Print and shaded views of the part. All mm, measured from the part's lowest x, y and z. Round coordinates to 2 decimals unless told otherwise and drop trailing zeros. Write each question's results on one line, items separated by ' | '. Start each with the question number.
1. Two-plate mould, pull along X, no slides. Class the marked faces 1, 2, 3 and 4: +X half, -X half, draft (parallel to the pull), parting line (faces both ways), or undercut.
2. Probe L1, parallel to Y at x = 2.5, z = 6; L2, parallel to X at y = 4.75, z = 9.5 (1 decimal); L3, parallel to Z at x = 7.5, y = 10.75 (1 decimal). List the from-to ranges inside material, lowest first. Write a range as [from, to].
3. Band-saw the part on A-A, the plane x = 5. Give the number of separate pieces and of enclosed holes in the cut face, then the cut area to 3 significant figures.
4. Drop flat-ended pins along their axis: pin 1 Ø4 at (x, y) = (5.5, 25.5) entering from -Z; pin 2 Ø1 at (x, z) = (5.5, 8.5) entering from +Y; pin 3 Ø3.5 at (x, y) = (5, 4.98) entering from -Z. Give the stop position or say it passes through.
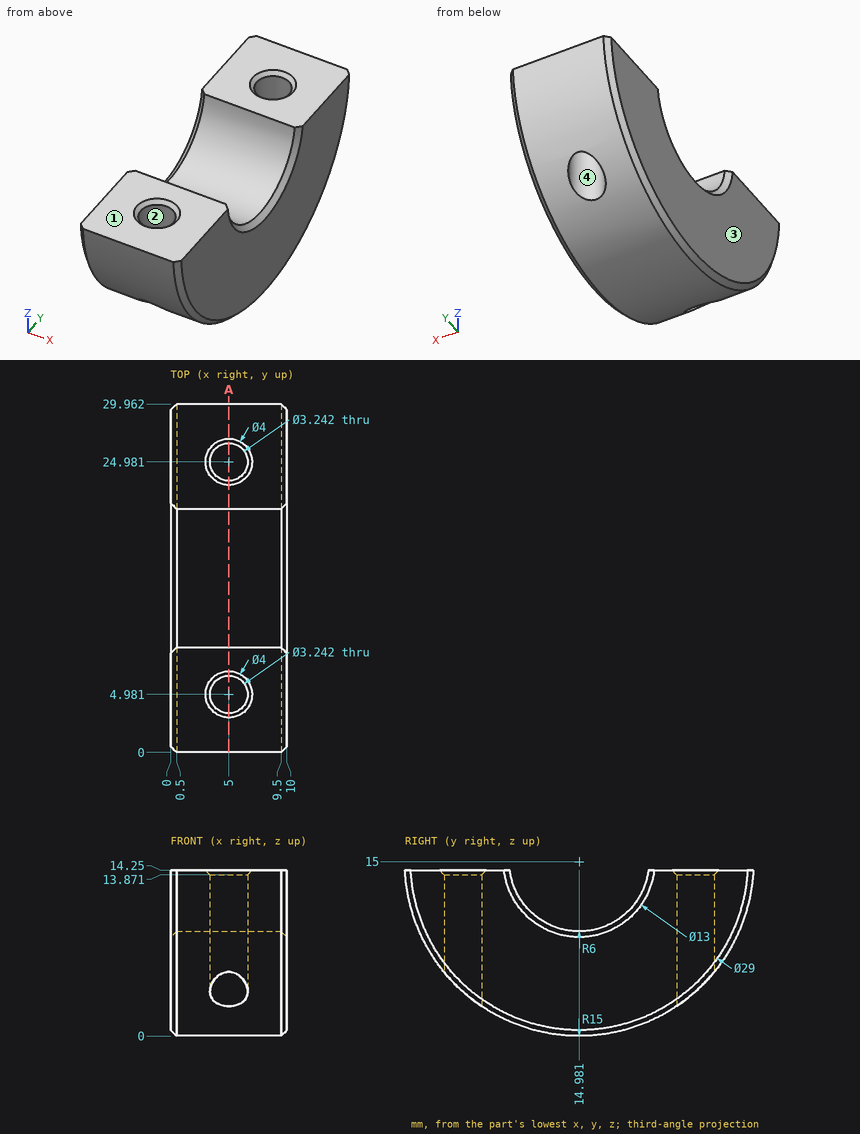
Solution:
1) face 1: draft | face 2: undercut | face 3: -X half | face 4: undercut
2) L1: [2.98, 26.98] | L2: [0, 3.4], [6.6, 10] | L3: [0.6, 10.7]
3) separate pieces: 3 | enclosed holes: 0 | area: 216 mm^2
4) pin 1: z = 2.66 | pin 2: y = 28.73 | pin 3: z = 2.47
